```python
from build123d import *

# Parameters (mm, degrees)
SKETCH1_W           = 45
SKETCH1_H           = 30
SKETCH1_R           = 1.5
BOSS_EXTRUDE1_DEPTH = 10
SKETCH5_W           = 13
SKETCH5_H           = 30
BOSS_EXTRUDE2_DEPTH = 28
SKETCH7_W           = 13
SKETCH7_H           = 8
CUT_EXTRUDE1_DEPTH  = 17
SKETCH8_R           = 1.5
CUT_EXTRUDE2_DEPTH  = 48.697863598
FILLET1_R           = 2


with BuildPart() as part:
    # Sketch1 → Boss-Extrude1 (new body)
    with BuildSketch(Plane(origin=(0, 0, 0), x_dir=(1, 0, 0), z_dir=(0, 1, 0))):
        with Locations((2.00430517, -0.186349789)):
            Rectangle(SKETCH1_W, SKETCH1_H)
        with Locations(Location((-7.99569483, 9.813650211, 0), (0, 0, 270))):
            Circle(SKETCH1_R, mode=Mode.SUBTRACT)
        with Locations(Location((12.00430517, 9.813650211, 0), (0, 0, 270))):
            Circle(SKETCH1_R, mode=Mode.SUBTRACT)
        with Locations(Location((12.00430517, -10.186349789, 0), (0, 0, 270))):
            Circle(SKETCH1_R, mode=Mode.SUBTRACT)
        with Locations(Location((-7.99569483, -10.186349789, 0), (0, 0, 270))):
            Circle(SKETCH1_R, mode=Mode.SUBTRACT)
    extrude(amount=-BOSS_EXTRUDE1_DEPTH)

    # Sketch5 → Boss-Extrude2 (add)
    with BuildSketch(Plane.XZ.offset(10)):
        with Locations((2.00430517, 0.186349789)):
            Rectangle(SKETCH5_W, SKETCH5_H)
    extrude(amount=BOSS_EXTRUDE2_DEPTH)

    # Sketch7 → Cut-Extrude1 (cut)
    with BuildSketch(Plane(origin=(0, 0, -14.813650211), x_dir=(-1, 0, 0), z_dir=(0, 0, -1))):
        with Locations((-2.00430517, -29)):
            Rectangle(SKETCH7_W, SKETCH7_H)
        with Locations((-2.00430517, -19)):
            Rectangle(SKETCH7_W, SKETCH7_H)
    extrude(amount=-CUT_EXTRUDE1_DEPTH, mode=Mode.SUBTRACT)

    # Sketch8 → Cut-Extrude2 (cut, through all)
    with BuildSketch(Plane.XZ.offset(38)):
        with Locations(Location((2.00430517, -8.813650211, 0), (0, 0, 270))):
            Circle(SKETCH8_R)
    extrude(amount=-CUT_EXTRUDE2_DEPTH, mode=Mode.SUBTRACT)

    # Fillet1
    fillet1_edges = [part.edges().sort_by_distance(p)[0] for p in [
        (16.50430517, -10, 15.186349789),
        (16.50430517, -10, -14.813650211),
        (24.50430517, -10, 0.186349789),
        (-4.49569483, -24, 15.186349789),
        (-4.49569483, -35.5, -14.813650211),
        (8.50430517, -35.5, -14.813650211),
        (8.50430517, -24, 15.186349789),
        (-4.49569483, -38, 0.186349789),
        (2.00430517, -38, -14.813650211),
        (8.50430517, -38, 0.186349789),
        (-12.49569483, -10, -14.813650211),
        (-20.49569483, -10, 0.186349789),
        (8.50430517, -24, -14.813650211),
        (8.50430517, -12.5, -14.813650211),
        (-12.49569483, -10, 15.186349789),
        (-4.49569483, -24, -14.813650211),
        (-4.49569483, -12.5, -14.813650211),
    ]]
    fillet(fillet1_edges, radius=FILLET1_R)


solid = part.part
```
Here's how the part is built. I have some questions about the finished solid (model axes, mm). A direction names the side the tool comes from. Coordinates: 2 decimals unless noted, no trailing zeros. Write each loop counter-clockwise with the first axis right and the second up, starting at its lowest first coordinate (ties: lowest second). Pieces come first, ordered by that corner, then holes. Notation, with made-up numbers: (3, 30.5) -> (11, 30.5) arc R17 cw to (11, 56.5) -> close; hole circle Ø11 at (37, -16.5). An arc over 180 degrees is marked (long way). Use a Markdown table: item, result. Add a question column.
(1) If we section it at D-D, the plane x = -1.5: Write out the boundary of the cut face in (y, z).
(2) Please list where these lines run through material, in increasing order: line 1 (Y direction, x = 6, z = -6.5); line 2 (Z direction, x = -7, y = -5); line 3 (X direction, y = -34, z = 12.75).
(3) I'm going to push flat-ended pins straight in: P1, Ø2, axis at y = -14.5, z = -4.5, coming from the +X side; P2, Ø4, axis at x = -8, z = -9.81, coming from the -Y side; P3, Ø4, axis at x = 2, z = -8.81, coming from the +Y side; P4, Ø13, axis at y = -21, z = 2.5, coming from the -X side. Where does each tip first touch, or does it pass through?
(4) We'd pull the mould along Y, two halves only. Please class faces 1 (the flat face through (2, -9, 15.186)), 2 (the flat face through (2, -38, 1)), 3 (the flat face through (2, -33, -6)): +Y half, -Y half, draft (parallel to the pull), parting line (faces both ways), or undercut.
(5) For faces 4 (the flat face through (-12, -10, 0)), 5 (the flat face through (15, -10, 0)), 6 (the flat face through (2, -19, 2.186)), 7 (the cylindrical face through (-3.93, -24.01, -14.21)), 8 (the cylindrical face through (15.63, -9.4, -14.24)), which set-ups out of +Z, -Z, +X, -X, +Y, -Y let a thin tool reach every point of the face, with its end or its side?
(6) If we section it at C-C, the plane z = 6.75: Write out the boundary of the cut face in (x, y), and give its area (3 significant figures).
(7) If we section it at B-B, the plane y = -31.5: Write out the boundary of the cut face in (x, z).
(8) If we section it at A-A, the plane z = -4: Write out the boundary of the cut face in (x, y), and give its area (3 significant figures).
Outcome:
| question | item | result |
|---|---|---|
| 1 | outline | (-38, -12.81) arc R2 ccw to (-36, -14.81) -> (-33, -14.81) -> (-33, 2.19) -> (-25, 2.19) -> (-25, -14.81) -> (-23, -14.81) -> (-23, 2.19) -> (-15, 2.19) -> (-15, -14.81) -> (0, -14.81) -> (0, 15.19) -> (-38, 15.19) -> close |
| 2 | line 1 | y = -38 to -33, -25 to -23, -15 to 0 |
| 2 | line 2 | z = -14.81 to -10.94, -8.69 to 9.06, 11.31 to 15.19 |
| 2 | line 3 | x = -4.5 to 8.5 |
| 3 | P1 | stops at x = 8.5 |
| 3 | P2 | stops at y = -10 |
| 3 | P3 | stops at y = 0 |
| 3 | P4 | stops at x = -4.5 |
| 4 | face 1 | draft |
| 4 | face 2 | -Y half |
| 4 | face 3 | undercut |
| 5 | face 4 | +Z, -Z, -X, -Y |
| 5 | face 5 | +Z, -Z, +X, -Y |
| 5 | face 6 | -Z, +X, -X |
| 5 | face 7 | -Z, -X, -Y |
| 5 | face 8 | -Z, +X, -Y |
| 6 | outline | (-20.5, -8) arc R2 ccw to (-18.5, -10) -> (-4.5, -10) -> (-4.5, -36) arc R2 ccw to (-2.5, -38) -> (6.5, -38) arc R2 ccw to (8.5, -36) -> (8.5, -10) -> (22.5, -10) arc R2 ccw to (24.5, -8) -> (24.5, 0) -> (-20.5, 0) -> close |
| 6 | area | 811 mm^2 |
| 7 | outline | (-4.5, 2.19) -> (8.5, 2.19) -> (8.5, 13.19) arc R2 ccw to (6.5, 15.19) -> (-2.5, 15.19) arc R2 ccw to (-4.5, 13.19) -> close |
| 8 | outline | (-20.5, -8) arc R2 ccw to (-18.5, -10) -> (-4.5, -10) -> (-4.5, -15) -> (8.5, -15) -> (8.5, -10) -> (22.5, -10) arc R2 ccw to (24.5, -8) -> (24.5, 0) -> (-20.5, 0) -> close; (-4.5, -36) arc R2 ccw to (-2.5, -38) -> (6.5, -38) arc R2 ccw to (8.5, -36) -> (8.5, -33) -> (-4.5, -33) -> close; (-4.5, -25) -> (8.5, -25) -> (8.5, -23) -> (-4.5, -23) -> close |
| 8 | area | 603 mm^2 |
